CAD build for the part. Positions are in the model's coordinates, mm. A direction names the side the tool comes from. Coordinates: 2 decimals unless noted, no trailing zeros. Loops run counter-clockwise (first coordinate to the right, second up) from the corner with the lowest first, then second, coordinate; pieces in that order, holes last. Notation, with made-up numbers: (-33.75, 61.25) -> (-15.75, 61.25) arc R11 ccw to (-15.75, 66.25) -> close; hole circle Ø5 at (-34, -21). An arc over 180 degrees is marked (long way). Return JSON: item names as keys, results as strings. Group by question number.
(1) Saw through at B-B on z = 1.75. Write the cut outline in (x, y), then the cut area to 3 significant figures.
(2) Tool access for faces 1 (the face through (15.465, 5.285, 9.699)), 2 (the face through (16, 5, 5)), 3 (the face through (19.5, 12.6, 0.5)): list every direction of +Z, -Z, +X, -X, +Y, -Y with a clear straight run to the whole face (end or side of a thin tool).
(3) Probe L1, parallel to X at y = 1.75, z = 2.5; L2, parallel to X at y = 7.25, z = 5.5; L3, parallel to Y at x = 4.25, z = 9.75. List the from-to ranges inside material, lowest first.
(4) Saw through at C-C on z = 8.5. Write the cut outline in (x, y).
(5) Mould opens along X. For faces 4 (the face through (6.1, 0.5, 0.5)), 5 (the face through (7.62, 6.32, 7.03)), 6 (the face through (9.5, 1.2, 0.5)) say: pulls with the +X half, pulls with the -X half, needs draft (parallel to the pull), parting line crosses it, or undercut.
(6) Saw through at A-A on x = 15.75. Write the cut outline in (y, z), then the cut area to 3 significant figures.
(7) Flat gauge pins, fed straight in: pin 1 Ø2.5 at (x, y) = (5.5, 10) entering from +Z; pin 2 Ø1.5 at (x, z) = (16.5, 3.5) entering from -Y; pin 3 Ø0.6 at (y, z) = (1, 5) entering from +X. Where does each tip first touch, or does it go through?
```python
from build123d import *

# Parameters (mm, degrees)
PAD_DEPTH       = 10
SKETCH001_R     = 2.5
POCKET_DEPTH    = 5
FILLET_R        = 3
CHAMFER_SIZE    = 2
FILLET001_R     = 1
CHAMFER001_SIZE = 1
SKETCH003_R     = 1.5
POCKET001_DEPTH = 5
CHAMFER002_SIZE = 0.25


with BuildPart() as part:
    # Sketch → Pad (new body)
    with BuildSketch(Plane.XY):
        Polygon((0, 0), (0, 20), (20, 20), (20, 5), (10, 5), (10, 0), align=None)
    extrude(amount=PAD_DEPTH)

    # Sketch001 (on Face8 of Pad) → Pocket (cut)
    with BuildSketch(Plane.XY.offset(10)):
        with Locations((6.464466, 8.535534)):
            Circle(SKETCH001_R)
    extrude(amount=-POCKET_DEPTH, mode=Mode.SUBTRACT)

    # Fillet
    fillet_edges = [part.edges().sort_by_distance(p)[0] for p in [
        (10, 5, 5),
    ]]
    fillet(fillet_edges, radius=FILLET_R)

    # Chamfer
    chamfer_edges = [part.edges().sort_by_distance(p)[0] for p in [
        (0, 0, 5),
        (20, 5, 5),
        (20, 20, 5),
        (0, 20, 5),
    ]]
    chamfer(chamfer_edges, length=CHAMFER_SIZE)

    # Fillet001
    fillet001_edges = [part.edges().sort_by_distance(p)[0] for p in [
        (6, 0, 10),
        (1, 1, 10),
        (10, 1, 10),
        (0, 10, 10),
        (10.87868, 4.12132, 10),
        (1, 19, 10),
        (15.5, 5, 10),
        (10, 20, 10),
        (19, 6, 10),
        (19, 19, 10),
        (20, 12.5, 10),
        (3.964466, 8.535534, 10),
    ]]
    fillet(fillet001_edges, radius=FILLET001_R)

    # Chamfer001
    chamfer001_edges = [part.edges().sort_by_distance(p)[0] for p in [
        (15.5, 5, 0),
        (19, 6, 0),
        (10.87868, 4.12132, 0),
        (20, 12.5, 0),
        (10, 1, 0),
        (19, 19, 0),
        (6, 0, 0),
        (10, 20, 0),
        (1, 1, 0),
        (1, 19, 0),
        (0, 10, 0),
    ]]
    chamfer(chamfer001_edges, length=CHAMFER001_SIZE)

    # Sketch003 (on Face9 of Chamfer001) → Pocket001 (cut)
    with BuildSketch(Plane(origin=(0, 0, 0), x_dir=(1, 0, 0), z_dir=(0, 0, -1))):
        with Locations((6.464466, -8.535534)):
            Circle(SKETCH003_R)
    extrude(amount=-POCKET001_DEPTH, mode=Mode.SUBTRACT)

    # Chamfer002
    chamfer002_edges = [part.edges().sort_by_distance(p)[0] for p in [
        (4.964466, 8.535534, 0),
        (4.964466, 8.535534, 5),
    ]]
    chamfer(chamfer002_edges, length=CHAMFER002_SIZE)


solid = part.part
```
Geometry results:
{
 "1": {"outline": "(0, 2) -> (2, 0) -> (10, 0) -> (10, 2) arc R3 cw to (13, 5) -> (18, 5) -> (20, 7) -> (20, 18) -> (18, 20) -> (2, 20) -> (0, 18) -> close; hole circle Ø3 at (6.46, 8.54)", "area": "337 mm²"},
 "2": {"face 1": "+Z, +X, -Y", "face 2": "+Z, -Z, +X, -Y", "face 3": "-Z, +X, +Y, -Y"},
 "3": {"L1": "0.25 to 10", "L2": "0 to 4.32, 8.61 to 20", "L3": "0.34 to 6.76, 10.31 to 19.66"},
 "4": {"outline": "(0, 2) -> (2, 0) -> (10, 0) -> (10, 2) arc R3 cw to (13, 5) -> (18, 5) -> (20, 7) -> (20, 18) -> (18, 20) -> (2, 20) -> (0, 18) -> close; hole circle Ø5 at (6.46, 8.54)"},
 "5": {"face 4": "needs draft", "face 5": "undercut", "face 6": "pulls with the +X half"},
 "6": {"outline": "(5, 1) -> (6, 0) -> (19, 0) -> (20, 1) -> (20, 9) arc R1 ccw to (19, 10) -> (6, 10) arc R1 ccw to (5, 9) -> close", "area": "149 mm²"},
 "7": {"pin 1": "z = 9.87", "pin 2": "y = 5", "pin 3": "x = 10"}
}
